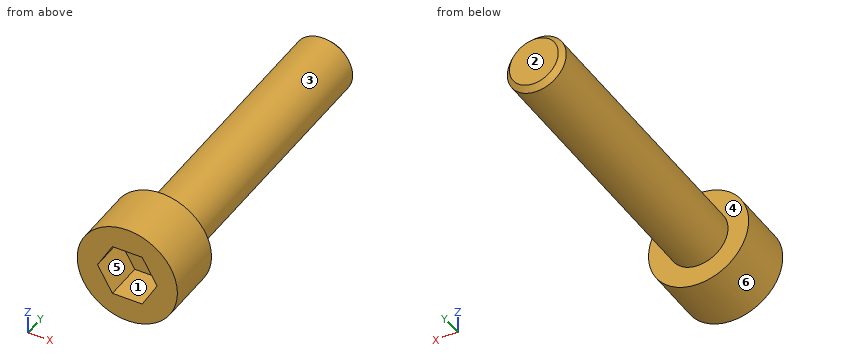
```python
from build123d import *

# Parameters (mm, degrees)
SKETCH1_R           = 2.465
BOSS_EXTRUDE1_DEPTH = 2.9
SKETCH2_R           = 1.45
BOSS_EXTRUDE2_DEPTH = 14
CUT_EXTRUDE1_DEPTH  = 1.9
CHAMFER1_SIZE       = 0.25


with BuildPart() as part:
    # Sketch1 → Boss-Extrude1 (new body)
    with BuildSketch(Plane(origin=(0, 0, 0), x_dir=(1, 0, 0), z_dir=(0, 1, 0))):
        Circle(SKETCH1_R)
    extrude(amount=BOSS_EXTRUDE1_DEPTH)

    # Sketch2 → Boss-Extrude2 (add)
    with BuildSketch(Plane(origin=(0, 2.9, 0), x_dir=(1, 0, 0), z_dir=(0, 1, 0))):
        Circle(SKETCH2_R)
    extrude(amount=BOSS_EXTRUDE2_DEPTH)

    # Sketch3 → Cut-Extrude1 (cut)
    with BuildSketch(Plane.XZ):
        Polygon((0.733234842, -1.27), (1.466469684, 0), (0.733234842, 1.27), (-0.733234842, 1.27), (-1.466469684, 0), (-0.733234842, -1.27), align=None)
    extrude(amount=-CUT_EXTRUDE1_DEPTH, mode=Mode.SUBTRACT)

    # Chamfer1
    chamfer1_edges = [part.edges().sort_by_distance(p)[0] for p in [
        (-1.45, 16.9, 0),
    ]]
    chamfer(chamfer1_edges, length=CHAMFER1_SIZE)


solid = part.part
```
Read the model definition and answer for the solid it produces. Units are mm, in the model's axes. Face numbers are marked on the shaded views. A direction names the side the tool comes from. Give positions to 0.01 mm unless a question says otherwise; leave off trailing zeros. Loops run counter-clockwise (first coordinate to the right, second up) from the corner with the lowest first, then second, coordinate; pieces in that order, holes last.
Item 1: The mould has two halves that part along X. Classify the marked faces 4, 5 and 6: released by +X, released by -X, zero draft, split by the parting line, or undercut.
Item 2: Find the intervals of material crossed by line 1 along Z through (x, y) = (-0.1, 5); line 2 along Y through (x, z) = (1.65, 0.15), in increasing order.
Item 3: Each of these flat-tipped pins is pushed along its axis until it touches: pin 1 Ø1.5 at (x, y) = (1.5, 3.5) entering from -Z; pin 2 Ø1 at (x, z) = (2, 0) entering from +Y; pin 3 Ø0.8 at (x, z) = (0, -0.5) entering from -Y. Where does it stop, or does it pass through?
Item 4: The part is cut by section D-D (x = 2.1). Write down the section's boundary in (y, z), and give its area (3 significant figures).
Item 5: For the marked faces 1, 2 and 3, determine the directions among +Z, -Z, +X, -X, +Y, -Y from which every point of the face is accessible in a straight line to the end or side of a thin tool.
Item 6: The part is cut by section B-B (y = 11.5). Write down the section's boundary in (x, z).
Item 7: The part is cut by section A-A (x = 0). Write down the section's boundary in (y, z) (3 decimals).
Item 8: The part is cut by section C-C (z = -1.9). Write down the section's boundary in (x, y).
Taken from the geometry:
1. face 4: zero draft
1. face 5: undercut
1. face 6: split by the parting line
2. line 1: z = -1.45 to 1.45
2. line 2: y = 0 to 2.9
3. pin 1: stops at z = -2.23
3. pin 2: stops at y = 2.9
3. pin 3: stops at y = 1.9
4. outline: (0, -1.29) - (2.9, -1.29) - (2.9, 1.29) - (0, 1.29) - close
4. area: 7.49 mm2
5. face 1: -Y
5. face 2: +Z, -Z, +X, -X, +Y
5. face 3: +Y
6. outline: circle Ø2.9 at (0, 0)
7. outline: (0, -2.465) - (2.9, -2.465) - (2.9, -1.45) - (16.65, -1.45) - (16.9, -1.2) - (16.9, 1.2) - (16.65, 1.45) - (2.9, 1.45) - (2.9, 2.465) - (0, 2.465) - (0, 1.27) - (1.9, 1.27) - (1.9, -1.27) - (0, -1.27) - close
8. outline: (-1.57, 0) - (1.57, 0) - (1.57, 2.9) - (-1.57, 2.9) - close
